Can you work these out from the drawing? Everything is in mm from the part's minimum corner. A direction names the side the tool comes from. Round coordinates to 2 decimals unless told otherwise and drop trailing zeros. Write each loop counter-clockwise with the first axis right and the second up, starting at its lowest first coordinate (ties: lowest second). Pieces come first, ordered by that corner, then holes. Notation, with made-up numbers: M 27.25,82 L 32.25,82 A21 cw 32.25,95 Z; hole C -37.75,25 d5. An arc over 180 degrees is marked long. Use one line per item in the form item = value. Start each with the question number.
Q1. I want a section at C-C on z = 28.5. List the corners of the cut face in (x, y) for me, and give its area (3 significant figures).
Q2. I'm going to push flat-ended pins straight in: pin 1 Ø0.6 at (y, z) = (23.5, 36.5) entering from -X; pin 2 Ø6 at (x, y) = (10.5, 15.5) entering from -Z; pin 3 Ø0.9 at (x, y) = (46.5, 5.5) entering from +Z. Where does each tip first touch, or does it pass through?
Q3. We'd pull the mould along Z, two halves only. Please class the marked faces 1, 2 and 3: +Z half, -Z half, draft (parallel to the pull), parting line (faces both ways), or undercut.
Q4. I want a section at B-B on y = 14. List the corners of the cut face in (x, z) for me, and give its area (3 significant figures).
Q5. I need wall thicknesses on line 1 along X through (y, z) = (9.5, 29.5); line 2 along Z through (x, y) = (42, 11.5); line 3 along Y through (x, z) = (44.5, 29). Which ranges of each line are inside material? Lowest first, please. Write a range as from..to.
Q6. I want a section at A-A on x = 23.5. List the corners of the cut face in (y, z) for me, and give its area (3 significant figures).
Q7. For the marked faces 4, 5 and 6, which set-ups out of +Z, -Z, +X, -X, +Y, -Y let a thin tool reach every point of the face, with its end or its side?
Q8. I want a section at D-D on x = 4.5. List the corners of the cut face in (y, z) for me, and give its area (3 significant figures).
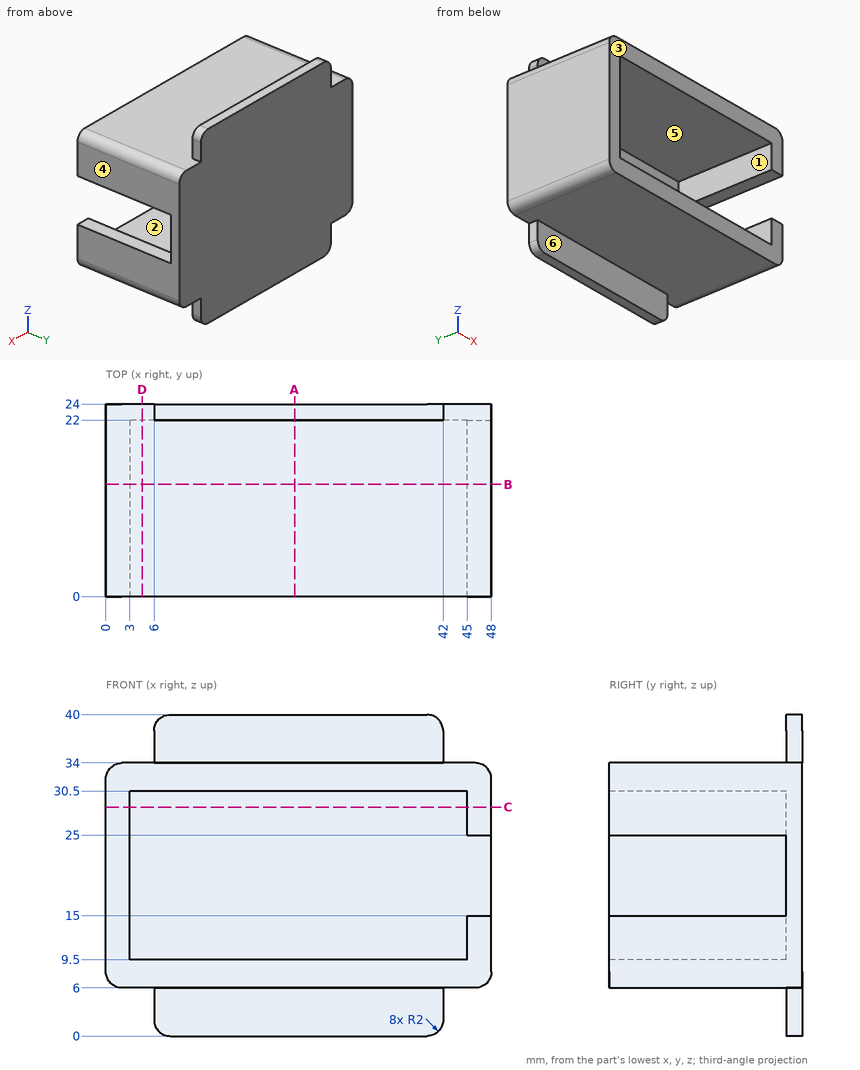
Reported:
q1.outline = M 0,0 L 3,0 L 3,22 L 45,22 L 45,0 L 48,0 L 48,24 L 0,24 Z
q1.area = 228 mm^2
q2.pin_1 = 6
q2.pin_2 = 6
q2.pin_3 = 34
q3.face_1 = undercut
q3.face_2 = undercut
q3.face_3 = draft
q4.outline = M 0,8 A2 ccw 2,6 L 46,6 A2 ccw 48,8 L 48,15 L 45,15 L 45,9.5 L 3,9.5 L 3,30.5 L 45,30.5 L 45,25 L 48,25 L 48,32 A2 ccw 46,34 L 2,34 A2 ccw 0,32 Z
q4.area = 429 mm^2
q5.line_1 = 0..3, 45..48
q5.line_2 = 6..9.5, 30.5..34
q5.line_3 = 22..24
q6.outline = M 0,6 L 22,6 L 22,0 L 24,0 L 24,40 L 22,40 L 22,34 L 0,34 L 0,30.5 L 22,30.5 L 22,9.5 L 0,9.5 Z
q6.area = 234 mm^2
q7.face_4 = +Z, -Z, +X, +Y, -Y
q7.face_5 = -Y
q7.face_6 = -Z, +X, -X, -Y
q8.outline = M 0,6 L 24,6 L 24,34 L 0,34 L 0,30.5 L 22,30.5 L 22,9.5 L 0,9.5 Z
q8.area = 210 mm^2
